from build123d import *
from OCP.BRepFilletAPI import BRepFilletAPI_MakeChamfer

# Parameters (mm, degrees)
SKETCH_1_R          = 25
SKETCH_1_R_2        = 21.5
EXTRUDE_1_DEPTH     = 10
SKETCH_2_W          = 6
SKETCH_2_H          = 20
EXTRUDE_2_DEPTH     = 58
SKETCH_3_W          = 15
SKETCH_3_H          = 20
EXTRUDE_3_DEPTH     = 10
SKETCH_4_R          = 2.3
CUT_EXTRUDE_1_DEPTH = 73.822129192
CHAMFER_2_SIZE      = 15.588457268
CHAMFER_2_SIZE_2    = 9
FILLET_1_R          = 3
SKETCH_5_R          = 4.3
CUT_EXTRUDE_2_DEPTH = 55
CHAMFER_3_SIZE      = 1
CHAMFER_3_SIZE2     = 1.732050808


with BuildPart() as part:
    # Sketch 1 → Extrude 1 (new body)
    with BuildSketch(Plane(origin=(0, 0, 0), x_dir=(1, 0, 0), z_dir=(0, 1, 0))):
        with Locations(Location((0, 0, 0), (0, 0, 270))):
            Circle(SKETCH_1_R)
        with Locations(Location((0, 0, 0), (0, 0, 270))):
            Circle(SKETCH_1_R_2, mode=Mode.SUBTRACT)
    extrude(amount=EXTRUDE_1_DEPTH)

    # Sketch 2 → Extrude 2 (add)
    with BuildSketch(Plane(origin=(0, 10, 0), x_dir=(-1, 0, 0), z_dir=(0, -1, 0))):
        with Locations((-24.25, 0)):
            Rectangle(SKETCH_2_W, SKETCH_2_H)
        with Locations((24.25, 0)):
            Rectangle(SKETCH_2_W, SKETCH_2_H)
    extrude(amount=EXTRUDE_2_DEPTH)

    # Sketch 3 → Extrude 3 (add)
    with BuildSketch(Plane.XZ.offset(48)):
        with Locations((28.75, 0)):
            Rectangle(SKETCH_3_W, SKETCH_3_H)
        with Locations((-28.75, 0)):
            Rectangle(SKETCH_3_W, SKETCH_3_H)
    extrude(amount=-EXTRUDE_3_DEPTH)

    # Sketch 4 → Cut-Extrude 1 (cut, through all)
    with BuildSketch(Plane.XZ.offset(48)):
        with Locations(Location((31, 0, 0), (0, 0, 270))):
            Circle(SKETCH_4_R)
        with Locations(Location((-31, 0, 0), (0, 0, 270))):
            Circle(SKETCH_4_R)
    extrude(amount=-CUT_EXTRUDE_1_DEPTH, mode=Mode.SUBTRACT)

    # Chamfer 2
    # the kernel refuses this chamfer: 15.588457268, 9 mm, written as the material it adds along each edge
    with BuildSketch(Plane(origin=(27.25, -38, 10), x_dir=(-0.01932676561270058, 0.9998132206222079, 0), z_dir=(0, 0, -1))) as chamfer_2_piece_1_section:
        Polygon((CHAMFER_2_SIZE * 0.99981322063, CHAMFER_2_SIZE * 0.0193267656128), (-CHAMFER_2_SIZE_2 * 0.0193267656127, CHAMFER_2_SIZE_2 * 0.999813220622), (0, 0), align=None)
    chamfer_2_piece_1 = extrude(amount=20, mode=Mode.PRIVATE)
    chamfer_2_piece_1 = split(chamfer_2_piece_1, bisect_by=Plane(origin=(36.25, -24.615994123, -6.666666667), z_dir=(-1, 0, 0)), keep=Keep.TOP, mode=Mode.PRIVATE)
    chamfer_2_piece_1 = chamfer_2_piece_1 - Plane(origin=(31, -24.615994123, 0), x_dir=(0, 0, -1), z_dir=(0, -1, 0)) * Cylinder(2.3, 103, mode=Mode.PRIVATE)
    add(chamfer_2_piece_1)
    with BuildSketch(Plane(origin=(-27.25, -38, -10), x_dir=(-0.9983227437537927, -0.0578938624026717, 0), z_dir=(0, 0, 1))) as chamfer_2_piece_2_section:
        Polygon((CHAMFER_2_SIZE_2 * 0.998322743754, -CHAMFER_2_SIZE_2 * 0.0578938624027), (-CHAMFER_2_SIZE * 0.0578938624031, -CHAMFER_2_SIZE * 0.998322743761), (0, 0), align=None)
    chamfer_2_piece_2 = extrude(amount=20, mode=Mode.PRIVATE)
    chamfer_2_piece_2 = split(chamfer_2_piece_2, bisect_by=Plane(origin=(-36.25, -35.368298987, 6.666666667), z_dir=(1, 0, 0)), keep=Keep.TOP, mode=Mode.PRIVATE)
    chamfer_2_piece_2 = chamfer_2_piece_2 - Plane(origin=(-31, -35.368298987, 0), x_dir=(0, 0, -1), z_dir=(0, -1, 0)) * Cylinder(2.3, 103, mode=Mode.PRIVATE)
    add(chamfer_2_piece_2)

    # Fillet 1
    fillet_1_edges = [part.edges().sort_by_distance(p)[0] for p in [
        (27.25, -6.205771366, -10),
        (27.25, -6.205771366, 10),
        (27.25, -22.411542732, 0),
        (-27.25, -6.205771366, -10),
        (-27.25, -6.205771366, 10),
        (-27.25, -22.411542732, 0),
        (31.75, -30.205771366, 10),
        (31.75, -30.205771366, -10),
        (-31.75, -30.205771366, 10),
        (-31.75, -30.205771366, -10),
        (0, 10, -25),
        (27.25, 10, 0),
        (21.25, -48, 0),
        (0, 10, 25),
        (-27.25, 10, 0),
        (-21.25, -48, 0),
    ]]
    fillet(fillet_1_edges, radius=FILLET_1_R)

    # Sketch 5 → Cut-Extrude 2 (cut)
    with BuildSketch(Plane(origin=(0, 10, 0), x_dir=(1, 0, 0), z_dir=(0, 1, 0))):
        with Locations(Location((31, 0, 0), (0, 0, 270))):
            Circle(SKETCH_5_R)
        with Locations(Location((-31, 0, 0), (0, 0, 321.134589702))):
            Circle(SKETCH_5_R)
    extrude(amount=-CUT_EXTRUDE_2_DEPTH, mode=Mode.SUBTRACT)

    # Chamfer 3: one chamfer whose edges measure the first distance from different faces: ONE call of the kernel's chamfer builder (chamfer() names one face for all edges)
    chamfer_3_edges_1 = [part.edges().sort_by_distance(p)[0] for p in [
        (0, 0, -21.5),
    ]]
    chamfer_3_side_1 = [part.faces().sort_by_distance(p)[0] for p in [
        (0, 5, -21.5),
    ]]
    chamfer_3_edges_2 = [part.edges().sort_by_distance(p)[0] for p in [
        (0, 0, 21.5),
    ]]
    chamfer_3_side_2 = [part.faces().sort_by_distance(p)[0] for p in [
        (0, 5, 21.5),
    ]]
    chamfer_3 = BRepFilletAPI_MakeChamfer(part.part.solid().wrapped)
    for e in chamfer_3_edges_1:
        chamfer_3.Add(CHAMFER_3_SIZE, CHAMFER_3_SIZE2, e.wrapped, chamfer_3_side_1[0].wrapped)  # the first distance lies on this face
    for e in chamfer_3_edges_2:
        chamfer_3.Add(CHAMFER_3_SIZE, CHAMFER_3_SIZE2, e.wrapped, chamfer_3_side_2[0].wrapped)  # the first distance lies on this face
    add(Compound.cast(chamfer_3.Shape()), mode=Mode.REPLACE)


solid = part.part
Model file for the job. Use its own axes, mm. A direction names the side the tool comes from. Give positions to 0.01 mm unless a question says otherwise; leave off trailing zeros. Order: outer loops, then holes, each group sorted by start corner. A loop starts at its lowest first (then second) coordinate and runs counter-clockwise, first axis right, second up. Notation, with made-up numbers: M 17,-14.5 L 67,-14.5 A25 ccw 67,17.5 Z; hole C 31.5,27.25 d10. An arc over 180 degrees is marked long. Put each result on its own line as item: value. Start each with the question number.
(1) Band-saw the part on A-A on y = -19. Give the cut face in (x, z).
(2) Pull direction Z, two halves, no side cores. Call faces 1 (the face through (-26, -32, 10)), 2 (the face through (28.755, -46.521, 0.499)), 3 (the face through (-31, -45, 3)), 4 (the face through (0, 3, -25)): released by +Z, released by -Z, zero draft, split by the parting line, or undercut.
(3) Drill centre lines: L1, parallel to X at y = -6, z = -4; L2, parallel to X at y = -47.3, z = 0; L3, parallel to X at y = -43, z = -5. Where is each one in solid material? Low to high. Write a range as [from, to].
(4) Band-saw the part on B-B on z = 0. Give the cut face in (x, y).
(5) Pin check, flat tips, straight feed: pin 1 Ø4.5 at (x, z) = (7.5, 19.5) entering from -Y; pin 2 Ø18.5 at (x, y) = (-32, -18) entering from -Z; pin 3 Ø18.5 at (x, y) = (-31, -5.5) entering from +Z. Stop position of each tip, or through.
(6) Tool access for faces 5 (the face through (-26.996, -29.699, 1.568)), 6 (the face through (-27.25, -7, -5)), 7 (the face through (26.39, -6.03, 9.1)): list every direction of +Z, -Z, +X, -X, +Y, -Y with a clear straight run to the whole face (end or side of a thin tool).
Results below:
1. outline: M -27.25,-7 A3 ccw -24.25,-10 L -21.25,-10 L -21.25,10 L -24.25,10 A3 ccw -27.25,7 L -27.25,2.1 A4.3 cw -27.25,-2.1 Z; M 21.25,-10 L 24.25,-10 A3 ccw 27.25,-7 L 27.25,-2.1 A4.3 cw 27.25,2.1 L 27.25,7 A3 ccw 24.25,10 L 21.25,10 Z
2. face 1: released by +Z
2. face 2: undercut
2. face 3: undercut
2. face 4: released by -Z
3. L1: x = [-27.25, -21.25], [21.25, 27.25]
3. L2: x = [-36.25, -33.3], [-28.7, -22.32], [22.32, 28.7], [33.3, 36.25]
3. L3: x = [-36.25, -21.25], [21.25, 36.25]
4. outline: M -36.25,-48 L -33.3,-48 L -33.3,-45 L -35.3,-45 L -35.3,-36.35 L -36.25,-38 Z; M -28.7,-48 L -24.25,-48 A3 ccw -21.25,-45 L -21.25,10 L -24.25,10 A3 ccw -26.7,8.73 L -26.7,-45 L -28.7,-45 Z; M 21.25,-45 A3 ccw 24.25,-48 L 28.7,-48 L 28.7,-45 L 26.7,-45 L 26.7,8.73 A3 ccw 24.25,10 L 21.25,10 Z; M 33.3,-48 L 36.25,-48 L 36.25,-38 L 35.3,-36.35 L 35.3,-45 L 33.3,-45 Z
5. pin 1: stops at y = 0.05
5. pin 2: stops at z = -10
5. pin 3: stops at z = 10
6. face 5: +Y
6. face 6: +Z, -Z, -X, +Y
6. face 7: +Z, +X, +Y
